Read the model definition and answer for the solid it produces. Units are mm, in the model's axes. A direction names the side the tool comes from. Round coordinates to 2 decimals unless told otherwise and drop trailing zeros. Write each loop counter-clockwise with the first axis right and the second up, starting at its lowest first coordinate (ties: lowest second). Pieces come first, ordered by that corner, then holes. Notation, with made-up numbers: (87.5, -33.5) - (123.5, -33.5) arc R28 cw to (123.5, -13.5) - close; hole circle Ø8 at (25, 34). An arc over 180 degrees is marked (long way). Use one line per item in the form item = value. Start each with the question number.
1) The part is cut by section A-A, the plane x = 274.5. Give the vertices of the cut face in (y, z), plus the area to 3 significant figures.
2) Each of these flat-tipped pins is pushed along its axis until it touches: pin 1 (12 mm diameter, centred on x = 477.5, z = 97.5, fed in from +Y); pin 2 (8 mm diameter, centred on x = 493, z = 157, fed in from +Y); pin 3 (6 mm diameter, centred on x = 275.5, z = 104, fed in from +Y). Where does it stop, or does it pass through?
3) Consider line 1 along Z through (x, y) = (791, 11); line 2 along Z through (x, y) = (150, -4.5); line 3 along Y through (x, z) = (148, 130). Determine where each line is inside the solid, lowest interval first. Write a range as from..to.
4) The part is cut by section B-B, the plane z = 42. Give the vertices of the cut face in (x, y).
5) For faces 5 (the face through (784.55, 20.56, 80.01)), 6 (the face through (451, 32, 20.433)), determine the directions among +Z, -Z, +X, -X, +Y, -Y from which every point of the face is accessible in a straight line to the end or side of a thin tool.
6) For a pull along X with two mould halves and no side action, classify faces 1 (the face through (754.001, 19.655, 98.781)), 2 (the face through (450.799, 33.085, 95.566)), 3 (the face through (0, 11, 64)), 4 (the face through (914.4, 11, 64)) as released by +X, released by -X, zero draft, split by the parting line, or undercut.
from build123d import *

# Parameters (mm, degrees)
BOSS_EXTRUDE1_DEPTH = 914.4
SKETCH6_R           = 33.902275387
CUT_EXTRUDE1_DEPTH  = 19.05


with BuildPart() as part:
    # Sketch1 → Boss-Extrude1 (new body)
    with BuildSketch(Plane(origin=(0, 0, 0), x_dir=(0, 0, -1), z_dir=(1, 0, 0))):
        Polygon((-20.432712568, 83.174071702), (-172.832712568, -18.425928298), (-20.432712568, -18.425928298), align=None)
    extrude(amount=BOSS_EXTRUDE1_DEPTH)

    # Sketch6 → Cut-Extrude1 (cut)
    with BuildSketch(Plane(origin=(0, 67.012532364, 44.675021576), x_dir=(1, 0, 0), z_dir=(0, 0.8320502943378435, 0.5547001962252294))):
        with Locations(Location((784.078611342, -55.644211071, 0), (0, 0, 270))):
            Circle(SKETCH6_R)
    extrude(amount=-CUT_EXTRUDE1_DEPTH, mode=Mode.SUBTRACT)


solid = part.part
Geometry results:
q1.outline = (-18.43, 20.43) - (83.17, 20.43) - (-18.43, 172.83) - close
q1.area = 7,740 mm2
q2.pin_1 = 35.8
q2.pin_2 = -5.2
q2.pin_3 = 29.46
q3.line_1 = 20.43..94.35, 114.1..128.69
q3.line_2 = 20.43..151.94
q3.line_3 = -18.43..10.13
q4.outline = (0, -18.43) - (914.4, -18.43) - (914.4, 68.8) - (0, 68.8) - close
q5.face_5 = none
q5.face_6 = -Z, +X, -X, +Y, -Y
q6.face_1 = undercut
q6.face_2 = zero draft
q6.face_3 = released by -X
q6.face_4 = released by +X
